Autodesk Inventor part; units mm, degrees
ref_plane "YZ Plane" through (0, 0, 0) normal (1, 0, 0) x (0, 1, 0)
ref_plane "XZ Plane" through (0, 0, 0) normal (0, 1, 0) x (-1, 0, 0)
ref_plane "XY Plane" through (0, 0, 0) normal (0, 0, 1) x (1, 0, 0)
sketch "Sketch1" plane through (0, 0, 0) normal (0, 0, 1) x (1, 0, 0)
  line L0 (0, 0) -> (127, 0)
  line L1 (127, 0) -> (127, 38.1)
  line L2 (127, 38.1) -> (0, 38.1)
  line L3 (0, 38.1) -> (0, 0)
  line L4 (0, 0) -> (16.129, 0)
  line L5 (127, 0) -> (110.871, 0)
  line L6 (16.129, 0) -> (16.129, 6.35)
  line L7 (16.129, 6.35) -> (0, 6.35)
  line L8 (110.871, 0) -> (110.871, 6.35)
  line L9 (110.871, 6.35) -> (127, 6.35)
  dimension "d0" = 127
  dimension "d1" = 38.1
  dimension "d2" = 16.129
  dimension "d3" = 16.129
  dimension "d4" = 6.35
  dimension "d5" = 6.35
extrude "Extrusion1" add sketch "Sketch1" along normal blind 76.2 contours L6 L7 L3 L2 L1 L9 L8 L0
chamfer "Chamfer5" distance 19.05 angle 60 1 edges at (127, 38.1, 38.1) measured on face at (127, 16.9333, 25.4)
chamfer "Chamfer6" distance 19.05 angle 60 1 edges at (0, 38.1, 38.1) measured on face at (0, 27.5167, 25.4)
sketch "Sketch8" plane through (127, 6.35, 76.2) normal (1, 0, 0) x (0, 0, -1)
  line L0 (0, 31.75) -> (0, 12.7)
  line L1 (0, 12.7) -> (12.7, 12.7)
  line L2 (0, 12.7) -> (76.2, 12.7)
  line L3 (12.7, 12.7) -> (12.7, 39.5471)
  line L4 (76.2, 12.7) -> (63.5, 12.7)
  line L5 (63.5, 12.7) -> (63.5, 39.5471)
  line L6 (12.7, 39.5471) -> (63.5, 39.5471)
  point P0 (76.2, -6.35)
  dimension "d37" = 12.7
  dimension "d38" = 12.7
extrude "Extrusion5" cut sketch "Sketch8" against normal blind 254
sketch "Sketch9" plane through (127, 19.05, 63.5) normal (0, 1, 0) x (1, 0, 0)
  line L0 (-127, 50.8) -> (-127, 0)
  line L1 (0, 0) -> (-127, 0)
  line L2 (0, 0) -> (0, 50.8)
  line L3 (0, 50.8) -> (-127, 50.8)
  line L4 (-94.0044, 50.8) -> (-32.9956, 50.8)
  line L5 (-63.5, 50.8) -> (-63.5, 0)
  circle A0 centre (-63.5, 25.4) radius 12.7
  point P0 (-127, 63.5)
  dimension "d41" = 25.4
extrude "Extrusion6" cut sketch "Sketch9" against normal blind 254 contours A0 L5 | L5 A0
properties part number "Block2" material "Stainless Steel"
Design review of the part built by this model. Coordinates are the model's own, in mm. A direction names the side the tool comes from. Coordinates: 2 decimals unless noted, no trailing zeros. Write each loop counter-clockwise with the first axis right and the second up, starting at its lowest first coordinate (ties: lowest second). Pieces come first, ordered by that corner, then holes. Notation, with made-up numbers: (30, 74) - (67, 74) arc R18 ccw to (67, 81) - close; hole circle Ø6 at (66.5, 71). An arc over 180 degrees is marked (long way). One line per item, written item: value.
1) Add section B-B (y = 29). State the section outline as (x, z) points.
Answer sheet:
outline: (17.23, 0) - (109.77, 0) - (109.77, 12.7) - (17.23, 12.7) - close; (17.23, 63.5) - (109.77, 63.5) - (109.77, 76.2) - (17.23, 76.2) - close
2) Add section D-D (x = 86). State the section outline as (y, z) points.
Answer sheet:
outline: (0, 0) - (38.1, 0) - (38.1, 12.7) - (19.05, 12.7) - (19.05, 63.5) - (38.1, 63.5) - (38.1, 76.2) - (0, 76.2) - close
3) Add section C-C (z = 23.5). State the section outline as (x, y) points.
Answer sheet:
outline: (0, 6.35) - (16.13, 6.35) - (16.13, 0) - (110.87, 0) - (110.87, 6.35) - (127, 6.35) - (127, 19.05) - (0, 19.05) - close
4) Mouldability with a two-part tool opening along Z and no side actions: class faces 1 (the face through (75.232, 9.658, 42.964)), 2 (the face through (110.27, 28.71, 6.44)), 3 (the face through (63, 19, 0)) as +Z half, -Z half, draft (parallel to the pull), parting line (faces both ways), or undercut.
Answer sheet:
face 1: undercut
face 2: draft
face 3: -Z half
5) For faces 4 (the face through (8, 6.35, 38)), 5 (the face through (63, 19, 76.2)), 6 (the face through (119, 6.35, 38)), 7 (the face through (64, 26, 63.5)), list the 3-axis set-ups (+Z, -Z, +X, -X, +Y, -Y) from which the entire face can be reached by the end or side of a thin tool; tool diameter is ignored.
Answer sheet:
face 4: +Z, -Z, -X, -Y
face 5: +Z, +X, -X, +Y, -Y
face 6: +Z, -Z, +X, -Y
face 7: +X, -X, +Y
6) Add section A-A (z = 38.1). State the section outline as (x, y) points, plus the area to 3 significant figures.
Answer sheet:
outline: (0, 6.35) - (16.13, 6.35) - (16.13, 0) - (50.8, 0) - (50.8, 19.05) - (0, 19.05) - close; (76.2, 0) - (110.87, 0) - (110.87, 6.35) - (127, 6.35) - (127, 19.05) - (76.2, 19.05) - close
area: 1,730 mm2
7) Insertion check: pin 1 (13 mm diameter, centred on x = 8.5, z = 36.5, fed in from -Y); pin 2 (1.9 mm diameter, centred on y = 4, z = 48.5, fed in from +X); pin 3 (5 mm diameter, centred on y = 2.5, z = 48.5, fed in from -X). Each pin has a flat end and moves straight along its axis. Give the tip position at first contact, or say it passes through.
Answer sheet:
pin 1: stops at y = 6.35
pin 2: stops at x = 110.87
pin 3: stops at x = 16.13
8) To check wall thickness, follow probe 1 along Z at (x, y) = (46, 22); probe 2 along Z at (x, y) = (63.5, 12); probe 3 along X at (y, z) = (4, 38). State the ranges of each line that lie inside material, in increasing order.
Answer sheet:
probe 1: z = 0 to 12.7, 63.5 to 76.2
probe 2: z = 0 to 25.4, 50.8 to 76.2
probe 3: x = 16.13 to 50.8, 76.2 to 110.87
